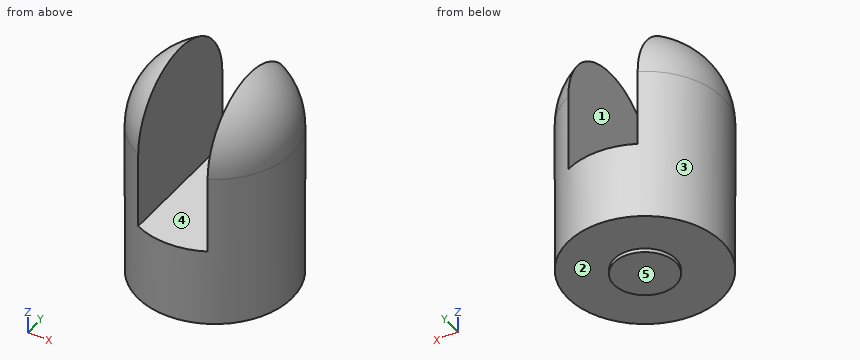
from build123d import *

# Parameters (mm, degrees)
SKETCH1_R           = 100
BOSS_EXTRUDE2_DEPTH = 200
DOME1_FACE_RADIUS   = 100
DOME1_HEIGHT        = 100
SKETCH3_W           = 90
SKETCH3_H           = 221.081096798
CUT_EXTRUDE1_DEPTH  = 200
SKETCH4_R           = 40
BOSS_EXTRUDE3_DEPTH = 5


with BuildPart() as part:
    # Sketch1 → Boss-Extrude2 (new body)
    with BuildSketch(Plane.XY):
        Circle(SKETCH1_R)
    extrude(amount=BOSS_EXTRUDE2_DEPTH)

    # Dome1: a dome of height H over a round flat face of radius A is a cap of a sphere of radius (A * A + H * H) / (2 * H)
    dome1_r = (DOME1_FACE_RADIUS * DOME1_FACE_RADIUS + DOME1_HEIGHT * DOME1_HEIGHT) / (2 * DOME1_HEIGHT)
    dome1_base = Plane((0, 0, 200), z_dir=(0, 0, 1))
    with Locations(dome1_base.offset(DOME1_HEIGHT - dome1_r)):
        dome1_ball = Sphere(dome1_r, mode=Mode.PRIVATE)
    add(split(dome1_ball, bisect_by=dome1_base, keep=Keep.TOP, mode=Mode.PRIVATE))

    # Sketch3 → Cut-Extrude1 (cut)
    with BuildSketch(Plane.XY.offset(300)):
        Rectangle(SKETCH3_W, SKETCH3_H)
    extrude(amount=-CUT_EXTRUDE1_DEPTH, mode=Mode.SUBTRACT)

    # Sketch4 → Boss-Extrude3 (add)
    with BuildSketch(Plane(origin=(0, 0, 0), x_dir=(-1, 0, 0), z_dir=(0, 0, -1))):
        Circle(SKETCH4_R)
    extrude(amount=BOSS_EXTRUDE3_DEPTH)


solid = part.part
Geometry: final body of the model. Coordinates: model frame, mm. Face numbers are marked on the shaded views. A direction names the side the tool comes from. Round coordinates to 2 decimals unless told otherwise and drop trailing zeros. Order: outer loops, then holes, each group sorted by start corner. A loop starts at its lowest first (then second) coordinate and runs counter-clockwise, first axis right, second up. Notation, with made-up numbers: (54, 68) -> (65, 68) arc R12 cw to (65, 91) -> close; hole circle Ø7 at (-25, 10.25). An arc over 180 degrees is marked (long way). Put each result on its own line as item: value. Start each with the question number.
Q1. Line query: probe 1 along Z at (x, y) = (34.5, 77.5); probe 2 along Z at (x, y) = (0.5, -29.5); probe 3 along X at (y, z) = (-59.5, 176.5). Output: solid intervals per line, ascending.
Q2. Section D-D on z = 52. Return the cut outline in (x, y), and give its area (3 significant figures).
Q3. Pull-direction query (X, two-part tool) for the marked faces 3, 4 and 5; classes: +X half, -X half, draft (parallel to the pull), parting line (faces both ways), or undercut.
Q4. Section A-A on y = 0. Return the cut outline in (x, z), and give its area (3 significant figures).
Q5. Reachability of the marked faces 1 and 2 from +Z, -Z, +X, -X, +Y, -Y: full face, straight path, thin tool, end or side. Return the list, or none.
Q6. Section C-C on z = 171. Return the cut outline in (x, y).
Q7. First-contact query: pin 1 (5 mm diameter, centred on y = -45.5, z = 211, fed in from +X); pin 2 (8 mm diameter, centred on x = 32, y = -56, fed in from -Z); pin 3 (4 mm diameter, centred on x = 76.5, z = 250, fed in from -Y). Flat tips, straight axial feed; report the tip coordinate or a pass-through.
Q8. Section B-B on x = 0. Return the cut outline in (y, z).
Ans:
1. probe 1: z = 0 to 100
1. probe 2: z = -5 to 100
1. probe 3: x = -80.37 to -45, 45 to 80.37
2. outline: circle Ø200 at (0, 0)
2. area: 31,400 mm2
3. face 3: parting line
3. face 4: undercut
3. face 5: draft
4. outline: (-100, 0) -> (-40, 0) -> (-40, -5) -> (40, -5) -> (40, 0) -> (100, 0) -> (100, 200) arc R100 ccw to (45, 289.3) -> (45, 100) -> (-45, 100) -> (-45, 289.3) arc R100 ccw to (-100, 200) -> close
4. area: 38,400 mm2
5. face 1: +Z, +Y, -Y
5. face 2: -Z
6. outline: (-45, -89.3) -> (-45, 89.3) arc R100 ccw to start; (45, -89.3) arc R100 ccw to (45, 89.3) -> close
7. pin 1: stops at x = 89.65
7. pin 2: stops at z = 0
7. pin 3: stops at y = -44.83
8. outline: (-100, 0) -> (-40, 0) -> (-40, -5) -> (40, -5) -> (40, 0) -> (100, 0) -> (100, 100) -> (-100, 100) -> close
